Autodesk Inventor part; units mm, degrees
ref_plane "YZ Plane" through (0, 0, 0) normal (1, 0, 0) x (0, 1, 0)
ref_plane "XZ Plane" through (0, 0, 0) normal (0, 1, 0) x (-1, 0, 0)
ref_plane "XY Plane" through (0, 0, 0) normal (0, 0, 1) x (1, 0, 0)
sketch "Sketch1" plane through (0, 0, 0) normal (0, 1, 0) x (-1, 0, 0)
  arc A0 (27.0056, -8.0993) -> (-27.0056, -8.0993) centre (0, 0) ccw
  line L0 (0, -43.942) -> (14.366, -43.942)
  line L1 (-14.366, -43.942) -> (0, -43.942)
  line L2 (0, 15.1299) -> (0, -95.843) construction
  line L3 (33.8234, 0) -> (-34.0336, 0) construction
  line L4 (16.256, 0) -> (16.256, -43.942) construction
  line L5 (16.7989, -42.1317) -> (27.0056, -8.0993)
  line L6 (-16.7989, -42.1317) -> (-27.0056, -8.0993)
  circle A1 centre (0, 0) radius 5.5372
  arc A2 (14.366, -43.942) -> (16.7989, -42.1317) centre (14.366, -41.402) ccw
  arc A3 (-16.7989, -42.1317) -> (-14.366, -43.942) centre (-14.366, -41.402) ccw
  circle A4 centre (7.9375, 0) radius 1.524
  line L7 (0, 0) -> (7.9375, 0) construction
  circle A5 centre (-7.9375, 0) radius 1.524
  line L8 (0, 0) -> (-7.9375, 0) construction
  circle A6 centre (16.256, 0) radius 1.524
  line L9 (0, 0) -> (16.256, 0) construction
  circle A7 centre (-16.256, 0) radius 1.524
  line L10 (0, 0) -> (-16.256, 0) construction
  circle A8 centre (23.0124, 0) radius 1.524
  line L11 (0, 0) -> (23.0124, 0) construction
  circle A9 centre (-23.0124, 0) radius 1.524
  line L12 (0, 0) -> (-23.0124, 0) construction
  point P0 (-16.256, -43.942)
  dimension "d0" = 56.388
  dimension "d4" = 16.256
  dimension "d5" = 16.256
  dimension "d6" = 43.942
  dimension "d7" = 11.0744
  dimension "d8" = 2.54
  dimension "d9" = 3.048
  dimension "d10" = 7.9375
  dimension "d12" = 3.048
  dimension "d13" = 16.256
  dimension "d15" = 3.048
  dimension "d16" = 23.0124
extrude "Extrusion1" add sketch "Sketch1" along normal blind 16.51
properties part number "encoder"
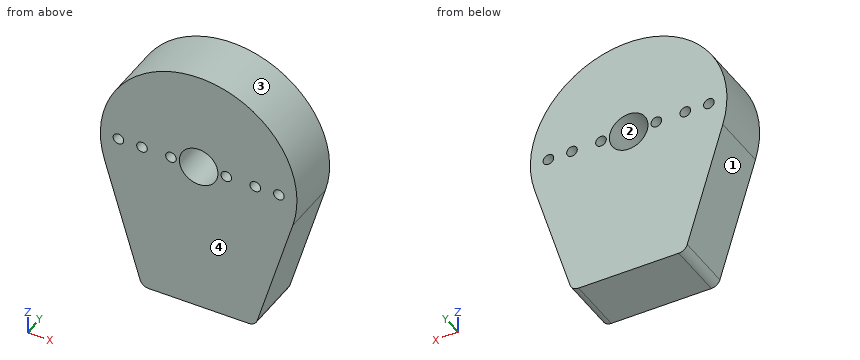
Build history of the part. All positions in model axes, mm. Face numbers are marked on the shaded views. Round coordinates to 2 decimals unless told otherwise and drop trailing zeros. Write each loop counter-clockwise with the first axis right and the second up, starting at its lowest first coordinate (ties: lowest second). Pieces come first, ordered by that corner, then holes. Notation, with made-up numbers: (54.5, 72.25) -> (91.5, 72.25) arc R29 cw to (91.5, 107.25) -> close; hole circle Ø3 at (46.25, 33). An arc over 180 degrees is marked (long way). Write item = value, one per line.
(1) Band-saw the part on A-A (x = 0). Give the cut face in (y, z).
Answer:
outline = (0, -43.94) -> (16.51, -43.94) -> (16.51, -5.54) -> (0, -5.54) -> close; (0, 5.54) -> (16.51, 5.54) -> (16.51, 28.19) -> (0, 28.19) -> close
(2) Band-saw the part on C-C (y = 4.75). Give the cut face in (x, z), then the cut area to 3 significant figures.
Answer:
outline = (-27.01, -8.1) -> (-16.8, -42.13) arc R2.54 ccw to (-14.37, -43.94) -> (14.37, -43.94) arc R2.54 ccw to (16.8, -42.13) -> (27.01, -8.1) arc R28.19 ccw (long way) to start; hole circle Ø3.05 at (-23.01, 0); hole circle Ø3.05 at (-16.26, 0); hole circle Ø3.05 at (-7.94, 0); hole circle Ø11.07 at (0, 0); hole circle Ø3.05 at (7.94, 0); hole circle Ø3.05 at (16.26, 0); hole circle Ø3.05 at (23.01, 0)
area = 3,110 mm2
(3) Probe L1, parallel to X at y = 10.5, z = 4; L2, parallel to Z at x = -7, y = 9.25; L3, parallel to X at y = 6.5, z = 5. List the from-to ranges inside material, lowest first.
Answer:
L1 = -27.91 to -3.83, 3.83 to 27.91
L2 = -43.94 to -1.2, 1.2 to 27.31
L3 = -27.75 to -2.38, 2.38 to 27.75
(4) Band-saw the part on B-B (z = 0). State how many separate pieces and enclosed holes the cut face has, then the cut area to 3 significant figures.
Answer:
separate_pieces = 8
enclosed_holes = 0
area = 446 mm2
(5) Two-plate mould, pull along X, no slides. Class the marked faces 1, 2, 3 and 4: pulls with the +X half, pulls with the -X half, needs draft (parallel to the pull), parting line crosses it, or undercut.
Answer:
face_1 = pulls with the -X half
face_2 = undercut
face_3 = parting line crosses it
face_4 = needs draft
(6) Flat gauge pins, fed straight in: pin 1 (5 mm diameter, centred on x = 7.94, z = 0, fed in from +Y); pin 2 (1.8 mm diameter, centred on x = 16.256, z = 0, fed in from +Y); pin 3 (8 mm diameter, centred on y = 6, z = -11.5, fed in from -X); pin 4 (3 mm diameter, centred on y = 6, z = -25.5, fed in from -X). Where does each tip first touch, or does it go through?
Answer:
pin_1 = 16.51
pin_2 = through
pin_3 = -27.18
pin_4 = -22.24
(7) Band-saw the part on D-D (x = -7.5). Give the cut face in (y, z), then the cut area to 3 significant figures.
Answer:
outline = (0, -43.94) -> (16.51, -43.94) -> (16.51, -1.46) -> (0, -1.46) -> close; (0, 1.46) -> (16.51, 1.46) -> (16.51, 27.18) -> (0, 27.18) -> close
area = 1,130 mm2
